from build123d import *

# Parameters (mm, degrees)
F0_R     = 2.54
F1_DEPTH = 8.89
F2_T     = -0.635
F3_W     = 3.81
F3_H     = 1.27
F4_DEPTH = 5.08


with BuildPart() as f1:
    # F0 (on Top) → F1 (new body)
    with BuildSketch(Plane.XY):
        Circle(F0_R)
    extrude(amount=F1_DEPTH)

    # F2
    f2_openings = [f1.faces().sort_by_distance(p)[0] for p in [
        (0, 0, 0),
    ]]
    offset(amount=F2_T, openings=f2_openings)

    # F3 (on face) → F4 (cut)
    with BuildSketch(Plane.XY.offset(8.89)):
        Rectangle(F3_W, F3_H)
    extrude(amount=-F4_DEPTH, mode=Mode.SUBTRACT)


solid = f1.part
Input: part model. Units: mm. Frame: model coordinates. A direction names the side the tool comes from. Round coordinates to 2 decimals unless told otherwise and drop trailing zeros. Write each loop counter-clockwise with the first axis right and the second up, starting at its lowest first coordinate (ties: lowest second). Pieces come first, ordered by that corner, then holes.
1) Cut plane A-A (x = 0). Return the cut outline in (y, z) (3 decimals).
2) Reachability of faces 1 (the cylindrical face through (-0.41, -1.86, 4.07)), 2 (the flat face through (1, 2, 0)), 3 (the flat face through (-0.01, 0.635, 8.43)) from +Z, -Z, +X, -X, +Y, -Y: full face, straight path, thin tool, end or side. Return the list, or none.
3) Ray query, L1, parallel to Y at x = 0, z = 2.25 (3 decimals); L2, parallel to Y at x = 0.55, z = 8.75 (3 decimals); L3, parallel to X at y = 1.65, z = 5. Return the intervals inside material, ascending.
4) Cut plane B-B (z = 5). Return the cut outline in (x, y) (3 decimals), then the cut area to 3 significant figures.
5) Draft query along Y for faces 4 (the flat face through (0, 1, 8.255)), 5 (the flat face through (0, -1, 8.89)), 6 (the cylindrical face through (-0.33, 2.52, 4.38)). Return one class per face: pulls with the +Y half, pulls with the -Y half, needs draft (parallel to the pull), parting line crosses it, or undercut.
6) Cut plane D-D (x = 1.2). Return the cut outline in (y, z) (3 decimals), then the cut area to 3 significant figures.
7) Contact query for flat-ended pins moving along their axis: P1, Ø0.6, axis at y = 0.5, z = 6, coming from the +X side; P2, Ø1, axis at x = 0.5, z = 1.5, coming from the +Y side. Output: stop coordinate, or through.
8) Cut plane C-C (y = -1.35). Return the cut outline in (x, z) (3 decimals), then the cut area to 3 significant figures.
Geometry says:
1. outline: (-2.54, 0) - (-1.905, 0) - (-1.905, 8.255) - (-0.635, 8.255) - (-0.635, 8.89) - (-2.54, 8.89) - close; (0.635, 8.255) - (1.905, 8.255) - (1.905, 0) - (2.54, 0) - (2.54, 8.89) - (0.635, 8.89) - close
2. face 1: -Z
2. face 2: -Z, +X, -X, +Y, -Y
2. face 3: +Z
3. L1: y = -2.54 to -1.905, 1.905 to 2.54
3. L2: y = -2.48 to -0.635, 0.635 to 2.48
3. L3: x = -1.93 to -0.95, 0.95 to 1.93
4. outline: circle Ø5.08 at (0, 0); hole (-1.905, -0.635) - (-1.796, -0.635) arc R1.905 ccw to (1.796, -0.635) - (1.905, -0.635) - (1.905, 0.635) - (1.796, 0.635) arc R1.905 ccw to (-1.796, 0.635) - (-1.905, 0.635) - close
4. area: 8.78 mm2
5. face 4: undercut
5. face 5: needs draft
5. face 6: parting line crosses it
6. outline: (-2.239, 0) - (-1.48, 0) - (-1.48, 8.255) - (-0.635, 8.255) - (-0.635, 8.89) - (-2.239, 8.89) - close; (0.635, 8.255) - (1.48, 8.255) - (1.48, 0) - (2.239, 0) - (2.239, 8.89) - (0.635, 8.89) - close
6. area: 14.6 mm2
7. P1: stops at x = 2.53
7. P2: stops at y = 2.54
8. outline: (-2.152, 0) - (-1.344, 0) - (-1.344, 8.255) - (1.344, 8.255) - (1.344, 0) - (2.152, 0) - (2.152, 8.89) - (-2.152, 8.89) - close
8. area: 16.1 mm2
